The model under review builds one solid part; all positions refer to its coordinate system, in mm. Face numbers are marked on the shaded views. A direction names the side the tool comes from. Round coordinates to 2 decimals unless told otherwise and drop trailing zeros. Loops run counter-clockwise (first coordinate to the right, second up) from the corner with the lowest first, then second, coordinate; pieces in that order, holes last. Notation, with made-up numbers: (84.25, -21) -> (118.25, -21) arc R14 ccw to (118.25, 1) -> close; hole circle Ø9 at (51, 56.25). An arc over 180 degrees is marked (long way). Use a Markdown table: item, result. Add a question column.
1) Consider section D-D on x = 12.75. Give the boundary of the cut face in (y, z) (3 decimals).
2) Consider section C-C on x = 2.5. Give the boundary of the cut face in (y, z), plus the area to 3 significant figures.
3) Consider section A-A on z = 0. Give the boundary of the cut face in (x, y) (3 decimals).
4) Wall thickness on probe 1 along Z at (x, y) = (11.5, -0.1); probe 2 along X at (y, z) = (0.7, 0.4); probe 3 along Y at (x, z) = (10.75, 0.8) (3 decimals): over which ranges is each line inside the solid? List them lowest first.
5) For the marked faces 1, 2 and 3, list the 3-axis set-ups (+Z, -Z, +X, -X, +Y, -Y) from which the entire face can be reached by the end or side of a thin tool; tool diameter is ignored.
6) Consider section B-B on y = 0. Give the boundary of the cut face in (x, z) (3 decimals).
7) Insertion check: pin 1 (0.6 mm diameter, centred on y = 1, z = -0.5, fed in from +X). The pin has a flat end and moves straight along its axis. Give the tip position at first contact, or say it passes through.
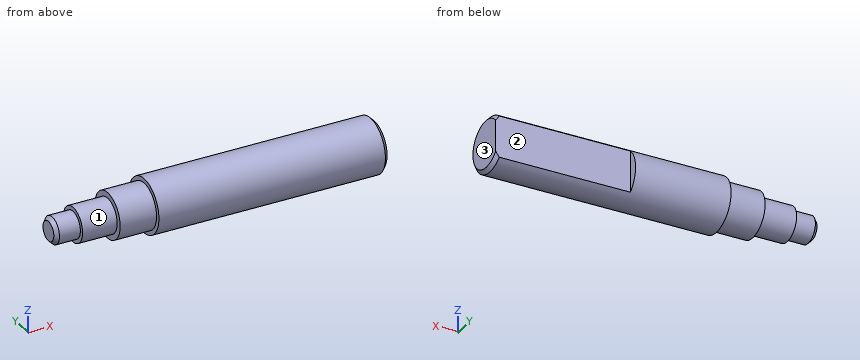
from build123d import *

# Parameters (mm, degrees)
CUT_EXTRUDE1_DEPTH = 7.4
CHAMFER1_SIZE      = 0.2


with BuildPart() as part:
    # Sketch1 → Revolve1 (revolve)
    with BuildSketch(Plane.XY, mode=Mode.PRIVATE) as revolve1_sk:
        Polygon((0, 0), (0, 0.735), (1.35, 0.735), (1.35, 0.95), (3.25, 0.95), (3.25, 1.25), (5.25, 1.25), (5.25, 1.485), (17.9, 1.485), (17.9, 0), align=None)
    revolve(revolve1_sk.sketch.rotate(Axis((-168.144085486, 0, 0), (1, 0, 0)), 90), axis=Axis((-168.144085486, 0, 0), (1, 0, 0)))

    # Sketch3 → Cut-Extrude1 (cut)
    with BuildSketch(Plane(origin=(17.9, 0, 0), x_dir=(0, 0, -1), z_dir=(1, 0, 0))):
        with BuildLine():
            Line((-1.128716085, 0.965), (1.128716085, 0.965))
            ThreePointArc((1.128716085, 0.965), (0, 1.485), (-1.128716085, 0.965))
        make_face()
    extrude(amount=-CUT_EXTRUDE1_DEPTH, mode=Mode.SUBTRACT)

    # Chamfer1
    chamfer1_edges = [part.edges().sort_by_distance(p)[0] for p in [
        (0, 0, -0.735),
        (17.9, -1.393084417, -0.514335306),
    ]]
    chamfer(chamfer1_edges, length=CHAMFER1_SIZE)


solid = part.part
Result set:
| question | item | result |
|---|---|---|
| 1 | outline | (0.965, -1.129) -> (0.965, 1.129) arc R1.485 ccw (long way) to start |
| 2 | outline | circle Ø1.9 at (0, 0) |
| 2 | area | 2.84 mm2 |
| 3 | outline | (0, -0.535) -> (0.2, -0.735) -> (1.35, -0.735) -> (1.35, -0.95) -> (3.25, -0.95) -> (3.25, -1.25) -> (5.25, -1.25) -> (5.25, -1.485) -> (17.7, -1.485) -> (17.9, -1.285) -> (17.9, 0.965) -> (10.5, 0.965) -> (10.5, 1.485) -> (5.25, 1.485) -> (5.25, 1.25) -> (3.25, 1.25) -> (3.25, 0.95) -> (1.35, 0.95) -> (1.35, 0.735) -> (0.2, 0.735) -> (0, 0.535) -> close |
| 4 | probe 1 | -1.48 to 1.48 |
| 4 | probe 2 | 1.35 to 17.9 |
| 4 | probe 3 | -1.251 to 0.965 |
| 5 | face 1 | -X |
| 5 | face 2 | +Z, -Z, +X, +Y |
| 5 | face 3 | +Z, -Z, +X, +Y, -Y |
| 6 | outline | (0, -0.535) -> (0.2, -0.735) -> (1.35, -0.735) -> (1.35, -0.95) -> (3.25, -0.95) -> (3.25, -1.25) -> (5.25, -1.25) -> (5.25, -1.485) -> (17.7, -1.485) -> (17.9, -1.285) -> (17.9, 1.285) -> (17.7, 1.485) -> (5.25, 1.485) -> (5.25, 1.25) -> (3.25, 1.25) -> (3.25, 0.95) -> (1.35, 0.95) -> (1.35, 0.735) -> (0.2, 0.735) -> (0, 0.535) -> close |
| 7 | pin 1 | x = 17.9 |
